For this review, take the finished solid that the model builds, in its own axes (mm). Face numbers are marked on the shaded views. A direction names the side the tool comes from. Give positions to 0.01 mm unless a question says otherwise; leave off trailing zeros. Write each loop counter-clockwise with the first axis right and the second up, starting at its lowest first coordinate (ties: lowest second). Pieces come first, ordered by that corner, then holes.
Q1. We need section A-A (x = 0). Write out the cut boundary in (y, z), then the cut area to 3 significant figures.
Q2. We need section D-D (z = -14.5). Write out the cut boundary in (x, y).
Q3. We need section B-B (z = 0). Write out the cut boundary in (x, y).
Q4. We need section C-C (y = 56). Write out the cut boundary in (x, z).
Q5. For line 1 (Y direction, x = -10.5, z = 6); line 2 (Z direction, x = 3, y = 26), list the stretches that pass through material, from the lowest coordinate up.
Q6. Insertion check: P1, Ø2, axis at y = 92, z = -3.5, coming from the -X side; P2, Ø2, axis at y = 50.5, z = -3, coming from the +X side; P3, Ø2, axis at x = -11, z = 7, coming from the +Y side; P4, Ø1, axis at y = 26, z = 11, coming from the -X side. Each pin has a flat end and moves straight along its axis. Give the tip position at first contact, or say it passes through.
Q7. Machinability: for the marked faces 1 and 2, which of the approach directions +Z, -Z, +X, -X, +Y, -Y give a long, thin tool a straight path to every point of the face, cutting with its end or side? Answer none if there is none.
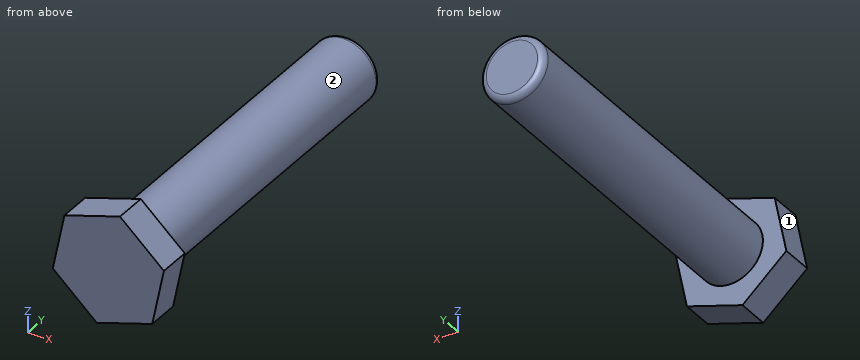
```python
from build123d import *

# Parameters (mm, degrees)
BOSS_EXTRU_1_DEPTH = 10
ESQUISSE2_R        = 10
BOSS_EXTRU_2_DEPTH = 105
CONG_1_R           = 2


with BuildPart() as part:
    # Esquisse1 → Boss.-Extru.1 (new body)
    with BuildSketch(Plane(origin=(0, 0, 0), x_dir=(1, 0, 0), z_dir=(0, 1, 0))):
        Polygon((-13.68952605, -12.09634845), (3.630982025, -17.90365155), (17.320508076, -5.807303101), (13.68952605, 12.09634845), (-3.630982025, 17.90365155), (-17.320508076, 5.807303101), align=None)
    extrude(amount=BOSS_EXTRU_1_DEPTH)

    # Esquisse2 → Boss.-Extru.2 (add)
    with BuildSketch(Plane(origin=(0, 10, 0), x_dir=(1, 0, 0), z_dir=(0, 1, 0))):
        Circle(ESQUISSE2_R)
    extrude(amount=BOSS_EXTRU_2_DEPTH)

    # Congé1
    cong_1_edges = [part.edges().sort_by_distance(p)[0] for p in [
        (-10, 115, 0),
    ]]
    fillet(cong_1_edges, radius=CONG_1_R)


solid = part.part
```
Computed:
1. outline: (0, -16.69) - (10, -16.69) - (10, -10) - (113, -10) arc R2 ccw to (115, -8) - (115, 8) arc R2 ccw to (113, 10) - (10, 10) - (10, 16.69) - (0, 16.69) - close
1. area: 2,430 mm2
2. outline: (-7.48, 0) - (6.52, 0) - (6.52, 10) - (-7.48, 10) - close
3. outline: (-16.14, 0) - (16.14, 0) - (16.14, 10) - (10, 10) - (10, 113) arc R2 ccw to (8, 115) - (-8, 115) arc R2 ccw to (-10, 113) - (-10, 10) - (-16.14, 10) - close
4. outline: circle Ø20 at (0, 0)
5. line 1: y = 0 to 10
5. line 2: z = -9.54 to 9.54
6. P1: stops at x = -9.68
6. P2: stops at x = 9.8
6. P3: stops at y = 10
6. P4: passes through
7. face 1: +Z, -X, +Y, -Y
7. face 2: +Y
